Source: CAD feature listing. Evaluate the final solid. Frame: model axes, mm. Round coordinates to 2 decimals unless told otherwise and drop trailing zeros. Loops run counter-clockwise (first coordinate to the right, second up) from the corner with the lowest first, then second, coordinate; pieces in that order, holes last. Notation, with made-up numbers: M -32,19 L 2,19 A19 ccw 2,37 Z; hole C -8,88.25 d2. An arc over 180 degrees is marked long. One line per item, written item: value.
Autodesk Inventor part; units mm, degrees
ref_plane "Arbeitsebene1" through (0, 0, -20) normal (0, 0, 1) x (1, 0, 0)
ref_plane "Arbeitsebene3" through (220, -220, -440) normal (-1, 0, 0) x (0, 0, 1)
ref_plane "YZ Plane" through (0, 0, 0) normal (1, 0, 0) x (0, 1, 0)
sketch "Skizze1" plane through (0, 0, 0) normal (0, 0, 1) x (1, 0, 0)
  line L0 (-220, -220) -> (220, -220)
  line L1 (220, 220) -> (220, -220)
  line L2 (-220, 220) -> (-220, -220)
  line L3 (-220, 220) -> (220, 220)
  line L4 (200, 200) -> (-200, 200)
  line L5 (-200, 200) -> (-200, -200)
  line L6 (-200, -200) -> (200, -200)
  line L7 (200, -200) -> (200, 200)
  line L8 (220, -220) -> (-220, -220)
  line L9 (-220, -220) -> (-220, 220)
  line L10 (-220, 220) -> (220, 220)
  line L11 (220, 220) -> (220, -220)
  line L12 (200, -200) -> (-200, -200)
  line L13 (-200, -200) -> (-200, 200)
  line L14 (-200, 200) -> (200, 200)
  line L15 (200, 200) -> (200, -200)
  point P0 (0, 0)
extrude "Extrusion1" add sketch "Skizze1" against normal blind 18
ref_plane "Arbeitsebene1" through (0, 0, -20) normal (0, 0, 1) x (1, 0, 0)
sketch "Skizze3" plane through (0, 0, -20) normal (0, 0, 1) x (1, 0, 0)
  arc A0 (-205, 25.5) -> (-205, 4.5) centre (-205, 15) ccw
  arc A1 (-205, 25.5) -> (-205, 4.5) centre (-205, 15) ccw
  arc A2 (-205, -5.9522) -> (-205, -26.9522) centre (-205, -16.4522) ccw
  arc A3 (-205, -5.9522) -> (-205, -26.9522) centre (-205, -16.4522) ccw
  arc A4 (-205, -5.9522) -> (-205, -26.9522) centre (-205, -16.4522) ccw
  arc A5 (-205, -5.9522) -> (-205, -26.9522) centre (-205, -16.4522) ccw
  line L0 (-200, -26.9522) -> (-205, -26.9522)
  line L1 (-205, -5.9522) -> (-200, -5.9522)
  line L2 (-205, 4.5) -> (-200, 4.5)
  line L3 (-200, -200) -> (-200, 200)
  line L4 (-205, 25.5) -> (-200, 25.5)
  line L5 (-205, -5.9522) -> (-200, -5.9522)
  line L6 (-205, -26.9522) -> (-200, -26.9522)
  arc A6 (-205, 25.5) -> (-205, 4.5) centre (-205, 15) ccw
  arc A7 (-205, -5.9522) -> (-205, -26.9522) centre (-205, -16.4522) ccw
  point P0 (0, 0)
extrude "Extrusion2" cut sketch "Skizze3" along normal blind 17
sketch "Skizze5" plane through (0, 0, -20) normal (0, 0, 1) x (1, 0, 0)
  line L0 (-200, -26.9522) -> (-200, -200)
  line L1 (-200, -200) -> (200, -200)
  line L2 (200, -200) -> (200, 200)
  line L3 (-200, 200) -> (200, 200)
  line L4 (-200, -200) -> (200, -200)
  line L5 (200, -200) -> (200, 200)
  line L6 (200, 200) -> (-200, 200)
  line L7 (-200, 200) -> (-200, -200)
  line L8 (-190, -190) -> (190, -190)
  line L9 (190, -190) -> (190, 190)
  line L10 (190, 190) -> (-190, 190)
  line L11 (-190, 190) -> (-190, -190)
  point P0 (0, 0)
  dimension "d8" = 10
  dimension "d9" = 10
  dimension "d10" = 10
  dimension "d11" = 10
extrude "Extrusion3" add sketch "Skizze5" along normal blind 8
ref_plane "Arbeitsebene3" through (220, -220, -440) normal (-1, 0, 0) x (0, 0, 1)
sketch "Skizze6" plane through (220, -220, -440) normal (-1, 0, 0) x (0, 0, 1)
  arc A0 (425, 193.0478) -> (425, 214.0478) centre (425, 203.5478) ccw
  arc A1 (425, 224.5) -> (425, 245.5) centre (425, 235) ccw
  line L0 (425, 224.5) -> (422, 224.5)
  line L1 (422, 214.0478) -> (425, 214.0478)
  line L2 (425, 193.0478) -> (422, 193.0478)
  line L3 (422, 245.5) -> (425, 245.5)
  line L4 (422, 193.0478) -> (428, 193.0478)
  line L5 (422, 193.0478) -> (425, 193.0478)
  line L6 (422, 214.0478) -> (425, 214.0478)
  line L7 (428, 214.0478) -> (422, 214.0478)
  line L8 (420, 245.5) -> (420, 224.5)
  line L9 (422, 224.5) -> (425, 224.5)
  line L10 (422, 245.5) -> (425, 245.5)
  line L11 (420, 193.0478) -> (420, 20)
  line L12 (422, 193.0478) -> (422, 214.0478)
  line L13 (422, 224.5) -> (422, 245.5)
  arc A2 (425, 193.0478) -> (425, 214.0478) centre (425, 203.5478) ccw
  arc A3 (425, 224.5) -> (425, 245.5) centre (425, 235) ccw
  point P0 (440, 220)
  point P1 (420, 20)
extrude "Extrusion4" cut sketch "Skizze6" along normal blind 25
sketch "Skizze7" plane through (0, 0, -20) normal (0, 0, -1) x (-1, 0, 0)
  line L0 (190, 190) -> (190, -190)
  line L1 (190, -190) -> (-190, -190)
  line L2 (-190, -190) -> (-190, 190)
  line L3 (-190, 190) -> (190, 190)
  line L4 (200, -200) -> (-200, -200)
  line L5 (200, 200) -> (200, -200)
  line L6 (-200, 200) -> (200, 200)
  line L7 (-200, -200) -> (-200, 200)
  line L8 (-200, 200) -> (200, 200)
  line L9 (-190, -190) -> (-190, 190)
  point P0 (0, 0)
extrude "Extrusion5" cut sketch "Skizze7" against normal blind 2
sketch "Skizze8" plane through (0, 0, -12) normal (0, 0, 1) x (1, 0, 0)
  line L0 (-200, -200) -> (200, -200)
  line L1 (200, -200) -> (200, 200)
  line L2 (200, 200) -> (-200, 200)
  line L3 (-200, 200) -> (-200, -200)
  line L4 (190, -190) -> (-190, -190)
  line L5 (-190, -190) -> (-190, 190)
  line L6 (-190, 190) -> (190, 190)
  line L7 (190, 190) -> (190, -190)
  line L8 (-200, -200) -> (200, -200)
  line L9 (200, -200) -> (200, 200)
  line L10 (200, 200) -> (-200, 200)
  line L11 (-200, 200) -> (-200, -200)
  point P0 (0, 0)
extrude "Extrusion6" add sketch "Skizze8" along normal blind 2
chamfer "Fase2" distance 18 angle 45 5 edges at (220, 122.75, -18) (220, -123.4761, -18) (220, -0.7261, -18) (0, 220, -18) (-220, 0, -18)
properties part number "PV_Ramen_CPY_3_CPY"
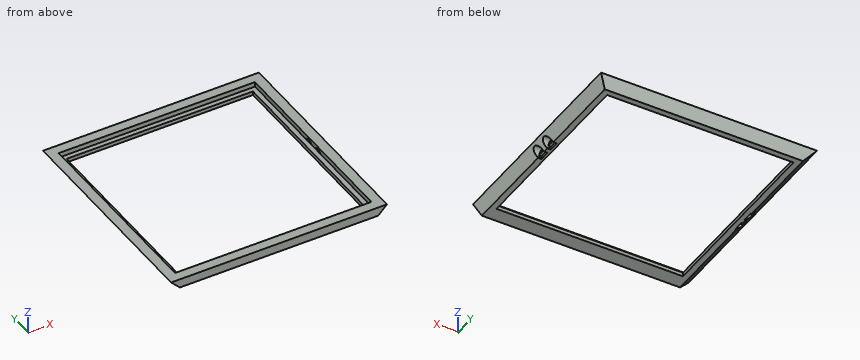
1. Section query A-A (y = -35). Return the cut outline in (x, z).
Report:
outline: M -220,0 L -202,-18 L -190,-18 L -190,-10 L -200,-10 L -200,0 Z; M 190,-18 L 202,-18 L 220,0 L 200,0 L 200,-10 L 190,-10 Z
2. Section query B-B (x = 139). Return the cut outline in (y, z).
Report:
outline: M -220,-18 L -190,-18 L -190,-10 L -200,-10 L -200,0 L -220,0 Z; M 190,-18 L 202,-18 L 220,0 L 200,0 L 200,-10 L 190,-10 Z
3. Pin query (flat end, axial travel): pin 1 (1.6 mm diameter, centred on y = 17, z = -11.5, fed in from +X); pin 2 (6.5 mm diameter, centred on y = -21.5, z = -15.5, fed in from +X); pin 3 (2.5 mm diameter, centred on x = 198.5, z = -16.5, fed in from +Y). Return the tip coordinate at first contact, or that it passes through.
Report:
pin 1: stops at x = 200
pin 2: stops at x = 195
pin 3: stops at y = 204.75
4. Ray query, line 1 (X direction, y = 134.5, z = -4.5); line 2 (X direction, y = 16, z = -15.25); line 3 (Y direction, x = 174, z = -15.5). Return the intervals inside material, ascending. Write a range as [from, to].
Report:
line 1: x = [-215.5, -200], [200, 215.5]
line 2: x = [-200, -190], [190, 195]
line 3: y = [-220, -190], [190, 204.5]
